from build123d import *

# Parameters (mm, degrees)
BOSS_EXTRUDE2_DEPTH = 1.524


with BuildPart() as part:
    # Sketch1 → Boss-Extrude2 (new body)
    with BuildSketch(Plane.XY):
        with BuildLine():
            Line((22.439190696, 2.281072115), (22.439190696, 15.440411119))
            Line((22.439190696, 15.440411119), (23.963190696, 15.440411119))
            Line((23.963190696, 15.440411119), (23.963190696, 2.281072115))
            ThreePointArc((23.963190696, 2.281072115), (24.875976359, 2.718444333), (25.496797873, 3.517852096))
            ThreePointArc((25.496797873, 3.517852096), (26.079485641, 4.314676532), (26.944327918, 4.790598847))
            ThreePointArc((26.944327918, 4.790598847), (27.306638474, 5.053990144), (27.391790825, 5.493754843))
            ThreePointArc((27.391790825, 5.493754843), (28.213802596, 6.77713145), (29.579242724, 7.454133758))
            ThreePointArc((29.579242724, 7.454133758), (30.268025744, 10.435749579), (29.751585716, 13.451996362))
            Line((29.751585716, 13.451996362), (28.227585716, 13.451996362))
            Line((28.227585716, 13.451996362), (28.227585716, 14.277496362))
            Line((28.227585716, 14.277496362), (26.703585716, 14.277496362))
            Line((26.703585716, 14.277496362), (26.703585716, 15.801496362))
            Line((26.703585716, 15.801496362), (28.227585716, 15.801496362))
            Line((28.227585716, 15.801496362), (28.227585716, 16.626996362))
            Line((28.227585716, 16.626996362), (29.751585716, 16.626996362))
            ThreePointArc((29.751585716, 16.626996362), (30.450938942, 17.551968079), (31.344559642, 18.290960401))
            ThreePointArc((31.344559642, 18.290960401), (31.016414864, 19.117764263), (30.611916517, 19.910017196))
            ThreePointArc((30.611916517, 19.910017196), (30.812764797, 20.413642259), (31.127845897, 20.854892911))
            ThreePointArc((31.127845897, 20.854892911), (30.608483418, 20.85451221), (30.117641351, 20.684772426))
            ThreePointArc((30.117641351, 20.684772426), (29.483865735, 21.483760637), (28.767611914, 22.209731818))
            ThreePointArc((28.767611914, 22.209731818), (28.825967468, 22.730638245), (28.945134545, 23.241077355))
            ThreePointArc((28.945134545, 23.241077355), (28.568640605, 22.947137357), (28.142874774, 22.730638245))
            ThreePointArc((28.142874774, 22.730638245), (27.099472832, 23.422587859), (25.973692104, 23.970401362))
            ThreePointArc((25.973692104, 23.970401362), (25.40453187, 24.652580061), (25.079145794, 25.479281369))
            ThreePointArc((25.079145794, 25.479281369), (24.923162133, 24.865841557), (24.450537029, 24.444813273))
            ThreePointArc((24.450537029, 24.444813273), (24.144286047, 24.507151138), (23.836139674, 24.559319007))
            ThreePointArc((23.836139674, 24.559319007), (23.336074732, 24.737274916), (22.998556028, 25.146926447))
            ThreePointArc((22.998556028, 25.146926447), (22.81061569, 24.832363061), (22.566241718, 24.559319007))
            ThreePointArc((22.566241718, 24.559319007), (22.258095346, 24.507151138), (21.951844363, 24.444813273))
            ThreePointArc((21.951844363, 24.444813273), (21.47921926, 24.865841557), (21.323235599, 25.479281369))
            ThreePointArc((21.323235599, 25.479281369), (20.997849523, 24.652580061), (20.428689288, 23.970401362))
            ThreePointArc((20.428689288, 23.970401362), (19.302908561, 23.422587859), (18.259506619, 22.730638245))
            ThreePointArc((18.259506619, 22.730638245), (17.833740787, 22.947137357), (17.457246848, 23.241077355))
            ThreePointArc((17.457246848, 23.241077355), (17.576413925, 22.730638245), (17.634769478, 22.209731818))
            ThreePointArc((17.634769478, 22.209731818), (16.918515657, 21.483760637), (16.284740042, 20.684772426))
            ThreePointArc((16.284740042, 20.684772426), (15.793897974, 20.85451221), (15.274535496, 20.854892911))
            ThreePointArc((15.274535496, 20.854892911), (15.589616595, 20.413642259), (15.790464876, 19.910017196))
            ThreePointArc((15.790464876, 19.910017196), (15.385966529, 19.117764263), (15.05782175, 18.290960401))
            ThreePointArc((15.05782175, 18.290960401), (15.951442451, 17.551968079), (16.650795677, 16.626996362))
            Line((16.650795677, 16.626996362), (18.174795677, 16.626996362))
            Line((18.174795677, 16.626996362), (18.174795677, 15.801496362))
            Line((18.174795677, 15.801496362), (19.698795677, 15.801496362))
            Line((19.698795677, 15.801496362), (19.698795677, 14.277496362))
            Line((19.698795677, 14.277496362), (18.174795677, 14.277496362))
            Line((18.174795677, 14.277496362), (18.174795677, 13.451996362))
            Line((18.174795677, 13.451996362), (16.650795677, 13.451996362))
            ThreePointArc((16.650795677, 13.451996362), (16.134355649, 10.435749579), (16.823138669, 7.454133758))
            ThreePointArc((16.823138669, 7.454133758), (18.188578797, 6.77713145), (19.010590568, 5.493754843))
            ThreePointArc((19.010590568, 5.493754843), (19.095742919, 5.053990144), (19.458053474, 4.790598847))
            ThreePointArc((19.458053474, 4.790598847), (20.322895752, 4.314676532), (20.905583519, 3.517852096))
            ThreePointArc((20.905583519, 3.517852096), (21.526405033, 2.718444333), (22.439190696, 2.281072115))
        make_face()
    extrude(amount=BOSS_EXTRUDE2_DEPTH)


solid = part.part
Here's how the part is built. I have some questions about the finished solid (model axes, mm). A direction names the side the tool comes from. Give positions to 0.01 mm unless a question says otherwise; leave off trailing zeros. Order: outer loops, then holes, each group sorted by start corner. A loop starts at its lowest first (then second) coordinate and runs counter-clockwise, first axis right, second up. Notation, with made-up numbers: (8.5, 50) -> (34.5, 50) arc R13 cw to (34.5, 65) -> close; hole circle Ø1 at (-23, 40.25). An arc over 180 degrees is marked (long way). Use a Markdown table: item, result. Add a question column.
Item 1: Imagine slicing it at A-A on y = 15. Please give me the cut outline in (x, z).
Item 2: I need wall thicknesses on line 1 (X direction, y = 10.75, z = 0.9); line 2 (X direction, y = 14.5, z = 0.85); line 3 (X direction, y = 16, z = 1.45). Which ranges of each line are inside material? Lowest first, please.
Item 3: Will these pins go through, and if not, where does the flat tip stop? pin 1 (0.8 mm diameter, centred on y = 15, z = 1, fed in from +X); pin 2 (0.5 mm diameter, centred on x = 17, z = 1, fed in from -Y); pin 3 (0.5 mm diameter, centred on x = 19, z = 0.5, fed in from +Y).
Item 4: Imagine slicing it at B-B on x = 28.5. Please give me the cut outline in (y, z), plus the area to 3 significant figures.
Item 5: For faces 1 (the face through (18.175, 14, 1)), 2 (the face through (15.801, 20.853, 0.751)), 3 (the face through (29, 16.627, 1)), 4 (the face through (22.439, 9, 1)), which set-ups out of +Z, -Z, +X, -X, +Y, -Y let a thin tool reach every point of the face, with its end or its side?
Item 6: If we mould it in two halves opening along Y, with no side actions, what happens to faces 5 (the face through (28.228, 16, 1)), 6 (the face through (28.57, 22.95, 0.75)), 7 (the face through (21.515, 2.727, 0.751))? For each: pulls with the +Y half, pulls with the -Y half, needs draft (parallel to the pull), parting line crosses it, or undercut.
Data:
| question | item | result |
|---|---|---|
| 1 | outline | (19.7, 0) -> (22.44, 0) -> (22.44, 1.52) -> (19.7, 1.52) -> close; (23.96, 0) -> (26.7, 0) -> (26.7, 1.52) -> (23.96, 1.52) -> close |
| 2 | line 1 | x = 16.13 to 22.44, 23.96 to 30.27 |
| 2 | line 2 | x = 19.7 to 22.44, 23.96 to 26.7 |
| 2 | line 3 | x = 18.17 to 28.23 |
| 3 | pin 1 | stops at x = 26.7 |
| 3 | pin 2 | stops at y = 7.34 |
| 3 | pin 3 | stops at y = 23.39 |
| 4 | outline | (7, 0) -> (13.45, 0) -> (13.45, 1.52) -> (7, 1.52) -> close; (16.63, 0) -> (22.91, 0) -> (22.91, 1.52) -> (16.63, 1.52) -> close |
| 4 | area | 19.4 mm² |
| 5 | face 1 | +Z, -Z, -X |
| 5 | face 2 | +Z, -Z, +Y |
| 5 | face 3 | +Z, -Z, +X |
| 5 | face 4 | +Z, -Z, -Y |
| 6 | face 5 | undercut |
| 6 | face 6 | pulls with the +Y half |
| 6 | face 7 | pulls with the -Y half |
